The listing builds one solid part. Answer for the finished solid, in the listing's coordinates (mm). A direction names the side the tool comes from. Coordinates: 2 decimals unless noted, no trailing zeros. Order: outer loops, then holes, each group sorted by start corner. A loop starts at its lowest first (then second) coordinate and runs counter-clockwise, first axis right, second up. Notation, with made-up numbers: (5, 75) -> (26, 75) arc R20 ccw to (26, 108) -> close; hole circle Ø6 at (40, -10.75). An arc over 180 degrees is marked (long way). Put each result on its own line as item: value. Start each with the question number.
```python
from build123d import *

# Parameters (mm, degrees)
BOSS_EXTRUDE1_DEPTH = 5
SKETCH2_R           = 2.1
SKETCH2_W           = 50
SKETCH2_H           = 5
CUT_EXTRUDE1_DEPTH  = 10
CUT_EXTRUDE2_DEPTH  = 10
CUT_EXTRUDE3_DEPTH  = 10
FILLET1_R           = 10
BOSS_EXTRUDE2_DEPTH = 5


with BuildPart() as part:
    # Sketch1 → Boss-Extrude1 (new body)
    with BuildSketch(Plane.XY):
        with BuildLine():
            Line((-10, 0), (-45, 0))
            ThreePointArc((-45, 0), (-52.071067812, 2.928932188), (-55, 10))
            Line((-55, 10), (-55, 100))
            ThreePointArc((-55, 100), (-90, 135), (-125, 100))
            Line((-125, 100), (-125, 10))
            ThreePointArc((-125, 10), (-127.928932188, 2.928932188), (-135, 0))
            Line((-135, 0), (-170, 0))
            ThreePointArc((-170, 0), (-177.071067812, 2.928932188), (-180, 10))
            Line((-180, 10), (-180, 175))
            ThreePointArc((-180, 175), (-178.535533906, 178.535533906), (-175, 180))
            Line((-175, 180), (-5, 180))
            ThreePointArc((-5, 180), (-1.464466094, 178.535533906), (0, 175))
            Line((0, 175), (0, 10))
            ThreePointArc((0, 10), (-2.928932188, 2.928932188), (-10, 0))
        make_face()
        with BuildLine():
            Line((-160, 175), (-10, 175))
            ThreePointArc((-10, 175), (-5, 170), (-10, 165))
            Line((-10, 165), (-160, 165))
            ThreePointArc((-160, 165), (-165, 170), (-160, 175))
        make_face(mode=Mode.SUBTRACT)
    extrude(amount=BOSS_EXTRUDE1_DEPTH)

    # Sketch2 → Cut-Extrude1 (cut)
    with BuildSketch(Plane.XY.offset(5)):
        with Locations((-135, 155)):
            Circle(SKETCH2_R)
        with Locations((-45, 155)):
            Circle(SKETCH2_R)
        with Locations((-90, 155)):
            Rectangle(SKETCH2_W, SKETCH2_H)
    extrude(amount=-CUT_EXTRUDE1_DEPTH, mode=Mode.SUBTRACT)

    # Sketch3 → Cut-Extrude2 (cut)
    with BuildSketch(Plane.XY.offset(5)):
        Polygon((0, 55), (0, 0), (-25, 0), align=None)
        Polygon((-155, 0), (-180, 55), (-180, 0), align=None)
    extrude(amount=-CUT_EXTRUDE2_DEPTH, mode=Mode.SUBTRACT)

    # Sketch4 → Cut-Extrude3 (cut)
    with BuildSketch(Plane.XY.offset(5)):
        Polygon((0, 155), (-10, 155), (-10, 33), (0, 55), align=None)
        Polygon((-180, 55), (-170, 33), (-170, 155), (-180, 155), align=None)
    extrude(amount=-CUT_EXTRUDE3_DEPTH, mode=Mode.SUBTRACT)

    # Fillet1
    fillet1_edges = [part.edges().sort_by_distance(p)[0] for p in [
        (0, 155, 2.5),
        (-180, 155, 2.5),
    ]]
    fillet(fillet1_edges, radius=FILLET1_R - 0.0001)  # a hair under: the kernel refuses the full size

    # Sketch5 → Boss-Extrude2 (add)
    with BuildSketch(Plane.XY.offset(5)):
        with BuildLine():
            Line((-10, 130), (-10, 110))
            ThreePointArc((-10, 110), (0, 120), (-10, 130))
        make_face()
    boss_extrude2 = extrude(amount=-BOSS_EXTRUDE2_DEPTH)

    # Mirror1: Boss-Extrude2 across plane
    add(boss_extrude2.mirror(Plane(origin=(-90, 0, 0), x_dir=(0, 0, 1), z_dir=(1, 0, 0))))


solid = part.part
```
(1) The part is cut by section A-A on x = -14. Determine the outline of the cut face in (y, z).
(2) Find the intervals of material crossed by L1, parallel to Y at x = -45, z = 1.65; L2, parallel to Y at x = -32, z = 2.85; L3, parallel to X at y = 92.5, z = 3.7, in increasing order.
(3) A tool of negligible diameter and unlimited length cuts with its end or side. For faces 1 (the cylindrical face through (-51.99, 2.85, 2.46)), 2 (the flat face through (-170, 71, 3)), 3 (the flat face through (-91, 180, 2)), 4 (the cylindrical face through (-3.01, 157.85, 2.46)), 5 (the cylindrical face through (-5, 170, 2)), from which of +Z, -Z, +X, -X, +Y, -Y can it reach the whole face along a straight path? Write none if from no direction.
(4) Each of these flat-tipped pins is pushed along its axis until it touches: P1, Ø2.5, axis at y = 146.5, z = 3.5, coming from the -X side; P2, Ø1.5, axis at x = -60, z = 3, coming from the -Y side; P3, Ø2.5, axis at x = -83.5, z = 1.5, coming from the -Y side. Where does it stop, or does it pass through?
(5) For a pull along X with two mould halves and no side action, classify faces 6 (the flat face through (-162.395, 16.269, 2.535)), 7 (the flat face through (-17.605, 16.269, 2.535)), 8 (the flat face through (-65, 155, 3)), 9 (the flat face through (-125, 56, 2)) as released by +X, released by -X, zero draft, split by the parting line, or undercut.
(6) The part is cut by section C-C on z = 3.65. Count the separate pieces of the cut face and the enclosed holes in it, plus the area to 3 significant figures.
(7) The part is cut by section B-B on y = 170. Determine the outline of the cut face in (x, z), plus the area to 3 significant figures.
(8) The part is cut by section D-D on x = -90. Determine the outline of the cut face in (y, z).
Worked out:
1. outline: (24.2, 0) -> (165, 0) -> (165, 5) -> (24.2, 5) -> close; (175, 0) -> (180, 0) -> (180, 5) -> (175, 5) -> close
2. L1: 0 to 152.9, 157.1 to 165, 175 to 180
2. L2: 0 to 165, 175 to 180
2. L3: -170 to -125, -55 to -10
3. face 1: +Z, -Z, -Y
3. face 2: +Z, -Z, -X, -Y
3. face 3: +Z, -Z, +X, -X, +Y
3. face 4: +Z, -Z, +X
3. face 5: +Z, -Z
4. P1: x = -170
4. P2: y = 116.72
4. P3: y = 134.13
5. face 6: released by -X
5. face 7: released by +X
5. face 8: undercut
5. face 9: undercut
6. separate pieces: 1
6. enclosed holes: 4
6. area: 18,200 mm2
7. outline: (-180, 0) -> (-165, 0) -> (-165, 5) -> (-180, 5) -> close; (-5, 0) -> (0, 0) -> (0, 5) -> (-5, 5) -> close
7. area: 100 mm2
8. outline: (135, 0) -> (152.5, 0) -> (152.5, 5) -> (135, 5) -> close; (157.5, 0) -> (165, 0) -> (165, 5) -> (157.5, 5) -> close; (175, 0) -> (180, 0) -> (180, 5) -> (175, 5) -> close
